Geometry check sheet. Reference: the model listing, model coordinates, mm. A direction names the side the tool comes from. Coordinates: 2 decimals unless noted, no trailing zeros. Order: outer loops, then holes, each group sorted by start corner. A loop starts at its lowest first (then second) coordinate and runs counter-clockwise, first axis right, second up. Notation, with made-up numbers: (84, 50) - (142, 50) arc R32 cw to (142, 80) - close; hole circle Ø2 at (-18.5, -35). An arc over 180 degrees is marked (long way). Put each result on its own line as item: value.
Autodesk Inventor part; units mm, degrees
ref_plane "YZ Plane" through (0, 0, 0) normal (1, 0, 0) x (0, 1, 0)
ref_plane "XZ Plane" through (0, 0, 0) normal (0, 1, 0) x (-1, 0, 0)
ref_plane "XY Plane" through (0, 0, 0) normal (0, 0, 1) x (1, 0, 0)
sketch "스케치1" plane through (0, 0, 0) normal (1, 0, 0) x (0, 1, 0)
  line L0 (0, 0) -> (5, 0)
  line L1 (5, 0) -> (5, 13)
  line L2 (5, 13) -> (0, 13)
  line L3 (0, 13) -> (0, 0)
  line L4 (0, 13) -> (7.5, 13)
  line L5 (7.5, 13) -> (7.5, 36)
  line L6 (7.5, 36) -> (0, 36)
  line L7 (0, 36) -> (0, 13)
  line L8 (0, 36) -> (10, 36)
  line L9 (10, 36) -> (10, 56)
  line L10 (10, 56) -> (0, 56)
  line L11 (0, 56) -> (0, 36)
  line L12 (0, 56) -> (7.5, 56)
  line L13 (7.5, 56) -> (7.5, 86)
  line L14 (7.5, 86) -> (0, 86)
  line L15 (0, 86) -> (0, 56)
  dimension "d0" = 10
  dimension "d1" = 15
  dimension "d2" = 20
  dimension "d3" = 15
  dimension "d4" = 13
  dimension "d5" = 23
  dimension "d6" = 20
  dimension "d7" = 30
revolve "회전1" add sketch "스케치1" angle 360 about axis through (0, 0, 36) along (0, 0, -1)
sketch "스케치2" plane through (0, 0, 0) normal (1, 0, 0) x (0, 1, 0)
  line L0 (5, 8.5) -> (5, 13)
  line L1 (5, 13) -> (3.85, 13)
  line L2 (3.85, 13) -> (3.85, 10.5)
  line L3 (3.85, 10.5) -> (5, 8.5)
  line L4 (-5, 13) -> (5, 13)
  line L5 (0, -17.2) -> (0, 103.2)
  point P0 (0, 0)
  dimension "d9" = 4.5
  dimension "d10" = 1.15
  dimension "d11" = 2.5
revolve "회전3" cut sketch "스케치2" angle 360 about axis through (0, 0, -10) along (0, 0, 1)
fillet "모깎기1" radius 0.8 2 edges at (0, -3.85, 10.5) (0, -3.85, 13)
thread "스레드1"
chamfer "모따기1" distance 1 angle 45 2 edges at (0, -5, 0) (0, -7.5, 86)
sketch "스케치3" plane through (0, 0, 0) normal (1, 0, 0) x (0, 1, 0)
  line L0 (11.8435, 67) -> (4.5, 67)
  line L1 (4.5, 67) -> (4.5, 82)
  line L2 (4.5, 82) -> (11.8435, 82)
  line L3 (11.8435, 82) -> (11.8435, 67)
  line L4 (-7.5, 86) -> (7.5, 86)
  line L5 (7.5, 86) -> (7.5, 56)
  point P0 (0, 0)
  dimension "d20" = 15
  dimension "d21" = 4
  dimension "d22" = 3
extrude "돌출1" cut sketch "스케치3" along normal mid plane 5
fillet "모깎기2" radius 2.5 4 edges at (2.5, 5.7855, 67) (-2.5, 5.7855, 67) (-2.5, 5.7855, 82) (2.5, 5.7855, 82)
fillet "모깎기3" radius 0.3 2 edges at (0, -7.5, 36) (0, -7.5, 56)
properties part number "3강 축1"
Q1. Thickness scan on L1, parallel to X at y = 0.5, z = 80.5; L2, parallel to Z at x = 1.5, y = -6; L3, parallel to Z at x = -1, y = 4.75. Record the ranges inside material, lowest first. Write a range as [from, to].
Answer block:
L1: x = [-7.48, 7.48]
L2: z = [13, 86]
L3: z = [0.85, 8.75], [13, 67.21], [81.79, 86]
Q2. Section check A-A on z = 25. Record the boundary of the cut face in (x, y), then the cut area to 3 significant figures.
Answer block:
outline: circle Ø15 at (0, 0)
area: 177 mm^2
Q3. Access from +Z, -Z, +X, -X, +Y, -Y to the whole of each face (thin tool, end or side, straight path). Record for faces 1 (the cylindrical face through (9.76, -2.17, 46.14)), 2 (the flat face through (-2.5, 6, 75)), 3 (the cylindrical face through (-3.76, -0.83, 11.45)), 4 (the cylindrical face through (-0.33, -7.493, 24.509)), 5 (the flat face through (-7.4, -3, 56)).
Answer block:
face 1: +Z, -Z
face 2: +Y
face 3: none
face 4: -Z
face 5: +Z
Q4. Draft check along X on faces 6 (the cylindrical face through (-0.33, -7.493, 70.851)), 7 (the flat face through (0, 0, 0)), 8 (the flat face through (2.5, 6, 75)). Enter one of: pulls with the +X half, pulls with the -X half, needs draft (parallel to the pull), parting line crosses it, or undercut.
Answer block:
face 6: parting line crosses it
face 7: needs draft
face 8: undercut
Q5. Section check B-B on z = 52. Record the boundary of the cut face in (x, y), then the cut area to 3 significant figures.
Answer block:
outline: circle Ø20 at (0, 0)
area: 314 mm^2
Q6. Depth check by flat-ended pin: pin 1 Ø1.5 at (x, y) = (7, 2) entering from +Z; pin 2 Ø1.3 at (y, z) = (5.5, 72.5) entering from +X; pin 3 Ø1.5 at (x, z) = (1, 76.5) entering from +Y. Enter the tip coordinate at first touch or a pass-through.
Answer block:
pin 1: stops at z = 85.97
pin 2: stops at x = 5.72
pin 3: stops at y = 4.5
